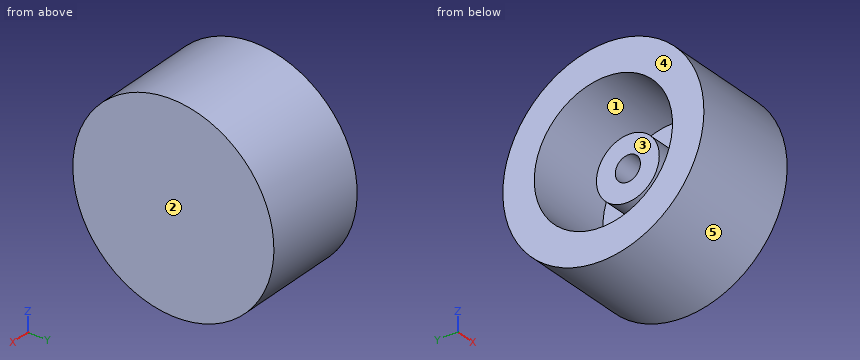
from build123d import *


with BuildPart() as part:
    # Esboço1 → Revolução1 (revolve)
    with BuildSketch(Plane.XY, mode=Mode.PRIVATE) as revolu_o1_sk:
        Polygon((0, 0), (0, 16), (-17, 16), (-17, 11), (-3, 11), (-3, 5), (-12, 5), (-12, 2), (-3, 2), (-3, 0), align=None)
    revolve(revolu_o1_sk.sketch.rotate(Axis((0, 0, 0), (-1, 0, 0)), 90), axis=Axis((0, 0, 0), (-1, 0, 0)))


solid = part.part
Read the model definition and answer for the solid it produces. Units are mm, in the model's axes. Face numbers are marked on the shaded views. A direction names the side the tool comes from. Round coordinates to 2 decimals unless told otherwise and drop trailing zeros. Order: outer loops, then holes, each group sorted by start corner. A loop starts at its lowest first (then second) coordinate and runs counter-clockwise, first axis right, second up.
1) Flat-ended cylindrical pins translate along their axes: pin 1 (4.5 mm diameter, centred on y = -1, z = -1, fed in from -X); pin 2 (1 mm diameter, centred on y = -6.5, z = 7, fed in from -X); pin 3 (1 mm diameter, centred on x = -15, y = -8.5, fed in from +Z). Find the tip coordinate at first contact, or state that the pin passes through.
2) The mould has two halves that part along Z. Classify the marked faces 3, 4 and 5: released by +Z, released by -Z, zero draft, split by the parting line, or undercut.
3) The part is cut by section B-B on y = 0. Write down the section's boundary in (x, z).
4) The part is cut by section A-A on x = -5.5. Write down the section's boundary in (y, z).
5) Straight lines are drawn through the part: L1, parallel to Y at x = -9, z = 0; L2, parallel to Y at x = -14, z = 0; L3, parallel to Z at x = -6.25, y = 1. For each, find the intervals that lie inside material, in ascending order.
6) The part is cut by section D-D on x = -12.5. Write down the section's boundary in (y, z), plus the area to 3 significant figures.
7) For the marked faces 1 and 2, determine the directions among +Z, -Z, +X, -X, +Y, -Y from which every point of the face is accessible in a straight line to the end or side of a thin tool.
Resolved:
1. pin 1: stops at x = -12
1. pin 2: stops at x = -3
1. pin 3: stops at z = 13.86
2. face 3: undercut
2. face 4: zero draft
2. face 5: split by the parting line
3. outline: (-17, -16) - (0, -16) - (0, 16) - (-17, 16) - (-17, 11) - (-3, 11) - (-3, 5) - (-12, 5) - (-12, 2) - (-3, 2) - (-3, -2) - (-12, -2) - (-12, -5) - (-3, -5) - (-3, -11) - (-17, -11) - close
4. outline: circle Ø32 at (0, 0); circle Ø10 at (0, 0); hole circle Ø22 at (0, 0); hole circle Ø4 at (0, 0)
5. L1: y = -16 to -11, -5 to -2, 2 to 5, 11 to 16
5. L2: y = -16 to -11, 11 to 16
5. L3: z = -15.97 to -10.95, -4.9 to -1.73, 1.73 to 4.9, 10.95 to 15.97
6. outline: circle Ø32 at (0, 0); hole circle Ø22 at (0, 0)
6. area: 424 mm2
7. face 1: -X
7. face 2: +Z, -Z, +X, +Y, -Y
